```python
from build123d import *

# Parameters (mm, degrees)
F1_DEPTH = 58
F3_START = -27
F2_W     = 105
F2_H     = 36
F3_DEPTH = 11
F4_R     = 3
F5_R     = 3
F7_DEPTH = 50


with BuildPart() as f1:
    # F0 (on Front) → F1 (new body)
    with BuildSketch(Plane.XZ):
        with BuildLine():
            Line((0, 9), (0, 0))
            Line((0, 0), (105, 0))
            Line((105, 0), (105, 9))
            Line((105, 9), (116, 9))
            ThreePointArc((116, 9), (102.5545593047, 29.883105595), (79.0811701161, 38))
            Line((79.0811701161, 38), (25.9188298839, 38))
            ThreePointArc((25.9188298839, 38), (2.4454406953, 29.883105595), (-11, 9))
            Line((-11, 9), (0, 9))
        make_face()
    extrude(amount=-F1_DEPTH)

    # F2 (on face) → F3 (cut)
    with BuildSketch(Plane(origin=(0, 0, 0), x_dir=(1, 0, 0), z_dir=(0, 0, -1)).offset(F3_START)):
        with Locations((52.5, -29)):
            Rectangle(F2_W, F2_H)
    extrude(amount=-F3_DEPTH, mode=Mode.SUBTRACT)

    # F4
    f4_edges = [f1.edges().sort_by_distance(p)[0] for p in [
        (102.554559, 58, 29.883106),
        (52.5, 58, 38),
        (2.445441, 58, 29.883106),
    ]]
    fillet(f4_edges, radius=F4_R)

    # F5
    f5_edges = [f1.edges().sort_by_distance(p)[0] for p in [
        (52.5, 0, 38),
        (2.445441, 0, 29.883106),
        (102.554559, 0, 29.883106),
    ]]
    fillet(f5_edges, radius=F5_R)

    # F6 (on face) → F7 (cut)
    with BuildSketch(Plane.XY.offset(27)):
        with BuildLine():
            Line((72, 23.3612143666), (91, 23.3612143666))
            ThreePointArc((91, 23.3612143666), (97.5, 29.8612143666), (91, 36.3612143666))
            Line((91, 36.3612143666), (72, 36.3612143666))
            ThreePointArc((72, 36.3612143666), (65.5, 29.8612143666), (72, 23.3612143666))
        make_face()
        with BuildLine():
            Line((33, 36.3612149123), (14, 36.3612149123))
            ThreePointArc((14, 36.3612149123), (7.5, 29.8612149123), (14, 23.3612149123))
            Line((14, 23.3612149123), (33, 23.3612149123))
            ThreePointArc((33, 23.3612149123), (39.5, 29.8612149123), (33, 36.3612149123))
        make_face()
    extrude(amount=-F7_DEPTH, mode=Mode.SUBTRACT)


solid = f1.part
```
Can you work these out from the model? Positions are in its coordinate system, mm. A direction names the side the tool comes from. Round coordinates to 2 decimals unless told otherwise and drop trailing zeros. Loops run counter-clockwise (first coordinate to the right, second up) from the corner with the lowest first, then second, coordinate; pieces in that order, holes last. Notation, with made-up numbers: M 77,-26.5 L 110,-26.5 A24 ccw 110,2.5 Z; hole C 31.5,-30 d7. An arc over 180 degrees is marked long. Answer in a Markdown table with one row per item.
1. If we section it at B-B, the plane y = 33: Please give me the cut outline in (x, z), plus the area to 3 significant figures.
Established:
| item | result |
|---|---|
| outline | M -11,9 L 0,9 L 0,0 L 8.31,0 L 8.31,27 L 0,27 L 0,27.79 A38 ccw Z; M 38.69,0 L 66.31,0 L 66.31,27 L 38.69,27 Z; M 96.69,0 L 105,0 L 105,9 L 116,9 A38 ccw 105,27.79 L 105,27 L 96.69,27 Z |
| area | 1,450 mm² |
2. On a 3-axis mill with a long thin cutter (end or side, diameter ignored), from which of +Z, -Z, +X, -X, +Y, -Y can I reach the whole of each face in a straight line? I mean faces 5 (the face through (39.5, 29.7, 13.7)), 6 (the face through (0, 29, 5)). Say none if no direction works.
Established:
| item | result |
|---|---|
| face 5 | +Z, -Z |
| face 6 | -Z, -X, +Y, -Y |
3. Please list where these lines run through material, in increasing order: line 1 (Y direction, x = 62, z = 28); line 2 (Y direction, x = 22, z = 23.5); line 3 (X direction, y = 54, z = 3.5). Write a range as from..to.
Established:
| item | result |
|---|---|
| line 1 | 0..11, 47..58 |
| line 2 | 0..23.36, 36.36..58 |
| line 3 | 0..105 |
4. Thinking about a two-plate mould opening in Y: for faces 1 (the face through (65.5, 30, 13.7)), 2 (the face through (110, 29, 9)), 3 (the face through (52.13, 0.86, 37.1)), 4 (the face through (82, 36.361, 14)), which applies, pulls with the +Y half, pulls with the -Y half, needs draft (parallel to the pull), parting line crosses it, or undercut?
Established:
| item | result |
|---|---|
| face 1 | undercut |
| face 2 | needs draft |
| face 3 | pulls with the -Y half |
| face 4 | undercut |
5. If we section it at A-A, the plane z = 4.5: Please give me the cut outline in (x, y).
Established:
| item | result |
|---|---|
| outline | M 0,0 L 105,0 L 105,58 L 0,58 Z; hole M 14,23.36 L 33,23.36 A6.5 ccw 33,36.36 L 14,36.36 A6.5 ccw Z; hole M 72,23.36 L 91,23.36 A6.5 ccw 91,36.36 L 72,36.36 A6.5 ccw Z |
6. I'm going to push flat-ended pins straight in: pin 1 Ø5.5 at (x, z) = (78.5, 14) entering from -Y; pin 2 Ø10 at (y, z) = (28, 2.5) entering from -X; pin 3 Ø10 at (y, z) = (16.5, 4.5) entering from +X; pin 4 Ø3 at (y, z) = (44.5, 24) entering from -X. Where does each tip first touch, or does it pass through?
Established:
| item | result |
|---|---|
| pin 1 | y = 0 |
| pin 2 | x = 0 |
| pin 3 | x = 116 |
| pin 4 | x = -4.7 |
